The model under review builds one solid part; all positions refer to its coordinate system, in mm. Coordinates: 2 decimals unless noted, no trailing zeros. Order: outer loops, then holes, each group sorted by start corner. A loop starts at its lowest first (then second) coordinate and runs counter-clockwise, first axis right, second up. Notation, with made-up numbers: (-10.5, 70) - (36.5, 70) arc R15 cw to (36.5, 95) - close; hole circle Ø1 at (57.5, 51.25). An arc over 180 degrees is marked (long way). Answer in a Markdown table with one row per item.
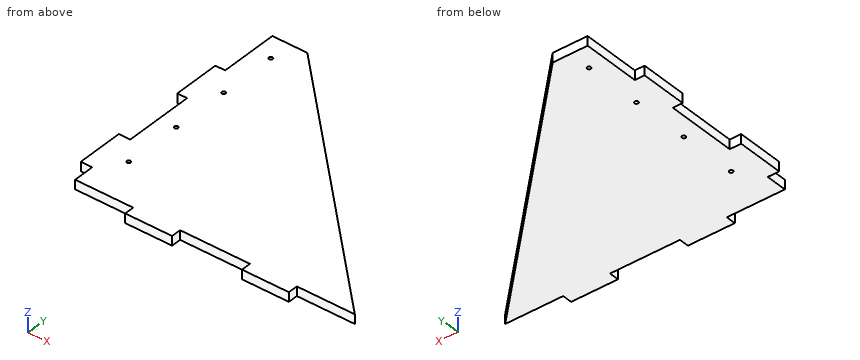
```python
from build123d import *

# Parameters (mm, degrees)
BOSS_EXTRUDE1_DEPTH = 4
SKETCH2_R           = 0.8
CUT_EXTRUDE1_DEPTH  = 4
LPATTERN1_COUNT     = 4
LPATTERN1_PITCH     = 25


with BuildPart() as part:
    # Sketch1 → Boss-Extrude1 (new body)
    with BuildSketch(Plane.XY):
        Polygon((0, 0), (0, 9.01), (-4.913167973, 9.01), (-4.913167973, 29.11), (0, 29.11), (0, 59.11), (-4.2, 59.11), (-4.2, 79.21), (0, 79.21), (0, 104.11), (15, 104.11), (120, 0), (95.1, 0), (95.1, -4.2), (75, -4.2), (75, 0), (45, 0), (45, -4.2), (24.9, -4.2), (24.9, 0), align=None)
    extrude(amount=BOSS_EXTRUDE1_DEPTH)

    # Sketch2 → Cut-Extrude1 (cut)
    with BuildSketch(Plane.XY.offset(4)):
        with Locations((7.5, 94.11)):
            Circle(SKETCH2_R)
    cut_extrude1 = extrude(amount=-CUT_EXTRUDE1_DEPTH, mode=Mode.SUBTRACT)

    # LPattern1: Cut-Extrude1 ×4
    with Locations(*[(0, -i * LPATTERN1_PITCH, 0) for i in range(1, LPATTERN1_COUNT)]):
        add(cut_extrude1, mode=Mode.SUBTRACT)


solid = part.part
```
Item 1: We need section A-A, the plane z = 1.7. Write out the cut boundary in (x, y), then the cut area to 3 significant figures.
Check values:
| item | result |
|---|---|
| outline | (-4.91, 9.01) - (0, 9.01) - (0, 0) - (24.9, 0) - (24.9, -4.2) - (45, -4.2) - (45, 0) - (75, 0) - (75, -4.2) - (95.1, -4.2) - (95.1, 0) - (120, 0) - (15, 104.11) - (0, 104.11) - (0, 79.21) - (-4.2, 79.21) - (-4.2, 59.11) - (0, 59.11) - (0, 29.11) - (-4.91, 29.11) - close; hole circle Ø1.6 at (7.5, 19.11); hole circle Ø1.6 at (7.5, 44.11); hole circle Ø1.6 at (7.5, 69.11); hole circle Ø1.6 at (7.5, 94.11) |
| area | 7,370 mm^2 |
Item 2: Clearance check with flat-ended pins moving along their axes: pin 1 Ø1.5 at (y, z) = (44.5, 2) entering from -X; pin 2 Ø1.2 at (x, z) = (-2.5, 3) entering from -Y; pin 3 Ø1.2 at (y, z) = (-2, 1) entering from -X; pin 4 Ø1.8 at (x, y) = (7.5, 94.11) entering from -Z. State where each tip first meets the part, or that it passes through.
Check values:
| item | result |
|---|---|
| pin 1 | x = 0 |
| pin 2 | y = 9.01 |
| pin 3 | x = 24.9 |
| pin 4 | z = 0 |
Item 3: We need section B-B, the plane x = 22. Write out the cut boundary in (y, z), then the cut area to 3 significant figures.
Check values:
| item | result |
|---|---|
| outline | (0, 0) - (97.17, 0) - (97.17, 4) - (0, 4) - close |
| area | 389 mm^2 |
Item 4: We need section C-C, the plane y = 87. Write out the cut boundary in (x, z), then the cut area to 3 significant figures.
Check values:
| item | result |
|---|---|
| outline | (0, 0) - (32.26, 0) - (32.26, 4) - (0, 4) - close |
| area | 129 mm^2 |
Item 5: To check wall thickness, follow line 1 (Y direction, x = 7.5, z = 2.85); line 2 (Y direction, x = 9, z = 0.45); line 3 (X direction, y = 94.11, z = 1.45). State the ranges of each line that lie inside material, in increasing order. Write a range as from..to.
Check values:
| item | result |
|---|---|
| line 1 | 0..18.31, 19.91..43.31, 44.91..68.31, 69.91..93.31, 94.91..104.11 |
| line 2 | 0..104.11 |
| line 3 | 0..6.7, 8.3..25.09 |
